For this review, use the dimensioned drawing (mm, ordinates from the lowest corner) and the shaded views. Round coordinates to 2 decimals unless told otherwise and drop trailing zeros. Loops run counter-clockwise (first coordinate to the right, second up) from the corner with the lowest first, then second, coordinate; pieces in that order, holes last. Notation, with made-up numbers: (-21, 53) - (26, 53) arc R21 cw to (26, 87) - close; hole circle Ø3 at (43.25, 35). An arc over 180 degrees is marked (long way). Use one line per item in the form item = value. Start each with the question number.
(1) We need section A-A, the plane y = 101.6. Write out the cut boundary in (x, z) (1 decimal), then the cut area to 3 significant figures.
(2) We need section D-D, the plane x = 231.5. Write out the cut boundary in (y, z), then the cut area to 3 significant figures.
(3) Wall thickness on probe 1 along Y at (x, z) = (101.6, 8.25) (1 decimal); probe 2 along X at (y, z) = (102.5, 5.25); probe 3 along Y at (x, z) = (219.5, 7): over which ranges is each line inside the solid? List them lowest first. Write a range as [from, to].
(4) We need section B-B, the plane x = 101.6. Write out the cut boundary in (y, z) (1 decimal), then the cut area to 3 significant figures.
(5) For pin 1 (2 mm diameter, centred on x = 129, z = 8, fed in from +Y); pin 2 (2 mm diameter, centred on x = 198, z = 9, fed in from +Y); pin 3 (1 mm diameter, centred on x = 157, z = 3.5, fed in from +Y), all flat-tipped, find the tip position at first contact; note any pin that passes through.
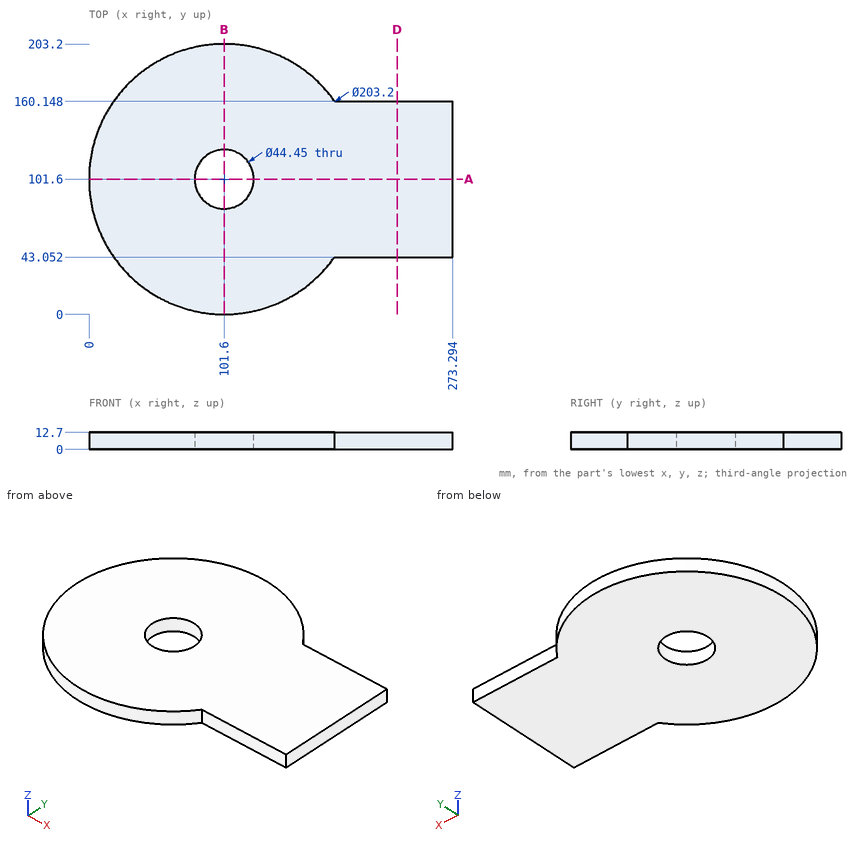
Data:
q1.outline = (0, 0) - (79.4, 0) - (79.4, 12.7) - (0, 12.7) - close; (123.8, 0) - (273.3, 0) - (273.3, 12.7) - (123.8, 12.7) - close
q1.area = 2,910 mm^2
q2.outline = (43.05, 0) - (160.15, 0) - (160.15, 12.7) - (43.05, 12.7) - close
q2.area = 1,490 mm^2
q3.probe_1 = [0, 79.4], [123.8, 203.2]
q3.probe_2 = [0, 79.39], [123.81, 273.29]
q3.probe_3 = [43.05, 160.15]
q4.outline = (0, 0) - (79.4, 0) - (79.4, 12.7) - (0, 12.7) - close; (123.8, 0) - (203.2, 0) - (203.2, 12.7) - (123.8, 12.7) - close
q4.area = 2,020 mm^2
q5.pin_1 = 199.71
q5.pin_2 = 160.15
q5.pin_3 = 187.09
